Geometry: final body of the model. Coordinates: model frame, mm. Face numbers are marked on the shaded views. A direction names the side the tool comes from. Round coordinates to 2 decimals unless told otherwise and drop trailing zeros. Loops run counter-clockwise (first coordinate to the right, second up) from the corner with the lowest first, then second, coordinate; pieces in that order, holes last. Notation, with made-up numbers: M 41,11 L 75,11 A31 cw 75,45 Z; hole C 48.5,54.5 d5. An arc over 180 degrees is marked long. Answer as a JSON object with one key per item and string values.
Autodesk Inventor part; units mm, degrees
ref_plane "YZ Plane" through (0, 0, 0) normal (1, 0, 0) x (0, 1, 0)
ref_plane "XZ Plane" through (0, 0, 0) normal (0, 1, 0) x (-1, 0, 0)
ref_plane "XY Plane" through (0, 0, 0) normal (0, 0, 1) x (1, 0, 0)
sketch "Skizze1" plane through (0, 0, 0) normal (0, 1, 0) x (-1, 0, 0)
  line L0 (-25, 25) -> (25, 25)
  line L1 (25, 25) -> (25, -25)
  line L2 (25, -25) -> (-25, -25)
  line L3 (-25, -25) -> (-25, 25)
  line L4 (-25, 25) -> (25, -25) construction
  line L5 (25, 25) -> (-25, -25) construction
  point P0 (0, 0)
  dimension "d0" = 50
  dimension "d1" = 50
extrude "Extrusion1" add sketch "Skizze1" along normal blind 6.5
sketch "Skizze2" plane through (0, 6.5, 0) normal (0, 1, 0) x (1, 0, 0)
  circle A0 centre (0, 0) radius 13.5
  dimension "d4" = 27
extrude "Extrusion2" add sketch "Skizze2" along normal blind 1.5
sketch "Skizze3" plane through (0, 8, 0) normal (0, 1, 0) x (1, 0, 0)
  circle A0 centre (0, 0) radius 13.5
hole "Bohrung1" at (0, 8, 0) direction (0, -1, 0) diameter 6.5 depth 8
sketch "Skizze4" plane through (0, 6.5, 0) normal (0, 1, 0) x (1, 0, 0)
  line L0 (25, -25) -> (25, 25)
  line L1 (25, 0) -> (-25, 0) construction
  line L2 (-25, 25) -> (-25, -25)
  line L3 (-25, -25) -> (25, -25)
  line L4 (0, -25) -> (0, 25) construction
  line L5 (25, 25) -> (-25, 25)
  point P0 (0, 0)
  point P1 (-21.124, 21.124)
  point P2 (-21.124, -21.124)
  point P3 (21.124, -21.124)
  point P4 (21.124, 21.124)
  dimension "d29" = 42.248
hole "Bohrung2" at (-21.124, 6.5, -21.124) at (-21.124, 6.5, 21.124) at (21.124, 6.5, 21.124) at (21.124, 6.5, -21.124) direction (0, -1, 0) diameter 6.5 depth 6.5
properties part number "cylinder_lid" material "Bronze, Guss"
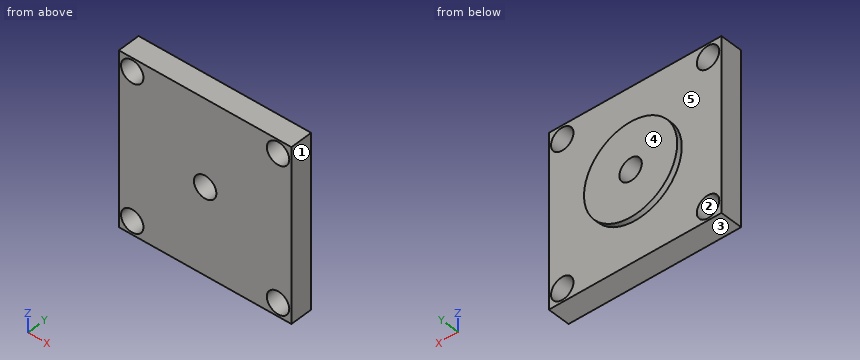
1) Section query C-C (z = 19.5). Return the cut outline in (x, y), and give its area (3 significant figures).
Results:
{"outline": "M -25,0 L -23.94,0 L -23.94,6.5 L -25,6.5 Z; M -18.31,0 L 18.31,0 L 18.31,6.5 L -18.31,6.5 Z; M 23.94,0 L 25,0 L 25,6.5 L 23.94,6.5 Z", "area": "252 mm2"}
2) Reachability of the marked faces 4 and 5 from +Z, -Z, +X, -X, +Y, -Y: full face, straight path, thin tool, end or side. Return the list, or none.
Results:
{"face 4": "+Z, -Z, +X, -X, +Y", "face 5": "+Y"}
3) Section query A-A (x = 0). Return the cut outline in (y, z).
Results:
{"outline": "M 0,-25 L 6.5,-25 L 6.5,-13.5 L 8,-13.5 L 8,-3.25 L 0,-3.25 Z; M 0,3.25 L 8,3.25 L 8,13.5 L 6.5,13.5 L 6.5,25 L 0,25 Z"}
4) Pull-direction query (X, two-part tool) for the marked faces 1, 2 and 3; classes: +X half, -X half, draft (parallel to the pull), parting line (faces both ways), or undercut.
Results:
{"face 1": "+X half", "face 2": "undercut", "face 3": "draft"}
5) Pin query (flat end, axial travel): P1, Ø7.5, axis at x = -21.124, z = 21.124, coming from the -Y side; P2, Ø6, axis at x = 0, z = 0, coming from the -Y side; P3, Ø1.5, axis at x = 9, z = 15, coming from the +Y side. Return the tip coordinate at first contact, or that it passes through.
Results:
{"P1": "y = 0", "P2": "through", "P3": "y = 6.5"}
6) Section query D-D (y = 7.25). Return the cut outline in (x, z).
Results:
{"outline": "C 0,0 d27; hole C 0,0 d6.5"}
7) Ray query, line 1 (X direction, y = 1.75, z = 21); line 2 (Z direction, x = -20, y = 3.25); line 3 (Y direction, x = 3, z = 20.5). Return the intervals inside material, ascending.
Results:
{"line 1": "-25 to -24.37, -17.88 to 17.88, 24.37 to 25", "line 2": "-25 to -24.17, -18.07 to 18.07, 24.17 to 25", "line 3": "0 to 6.5"}
8) Section query B-B (z = 0). Return the cut outline in (x, y).
Results:
{"outline": "M -25,0 L -3.25,0 L -3.25,8 L -13.5,8 L -13.5,6.5 L -25,6.5 Z; M 3.25,0 L 25,0 L 25,6.5 L 13.5,6.5 L 13.5,8 L 3.25,8 Z"}
